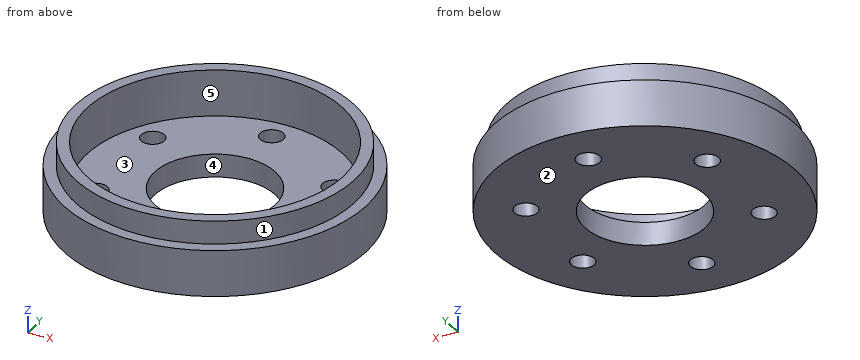
from build123d import *

# Parameters (mm, degrees)
SKETCH_1_R          = 32.5
SKETCH_1_R_2        = 13
EXTRUDE_1_DEPTH     = 5
SKETCH_2_R          = 32.5
SKETCH_2_R_2        = 27.5
EXTRUDE_2_DEPTH     = 5
SKETCH_3_R          = 2.5
CUT_EXTRUDE_1_DEPTH = 47.233105022
SKETCH_4_R          = 30
SKETCH_4_R_2        = 27.5
EXTRUDE_3_DEPTH     = 5


with BuildPart() as part:
    # 草图1 → 凸台-拉伸1 (new body)
    with BuildSketch(Plane.XY):
        Circle(SKETCH_1_R)
        Circle(SKETCH_1_R_2, mode=Mode.SUBTRACT)
    extrude(amount=EXTRUDE_1_DEPTH)

    # 草图2 → 凸台-拉伸2 (add)
    with BuildSketch(Plane.XY.offset(5)):
        Circle(SKETCH_2_R)
        Circle(SKETCH_2_R_2, mode=Mode.SUBTRACT)
    extrude(amount=EXTRUDE_2_DEPTH)

    # 草图3 → 切除-拉伸1 (cut, through all)
    with BuildSketch(Plane.XY.offset(5)):
        with Locations((0, 22.5)):
            Circle(SKETCH_3_R)
        with Locations((19.485571585, 11.25)):
            Circle(SKETCH_3_R)
        with Locations((19.485571585, -11.25)):
            Circle(SKETCH_3_R)
        with Locations((0, -22.5)):
            Circle(SKETCH_3_R)
        with Locations((-19.485571585, -11.25)):
            Circle(SKETCH_3_R)
        with Locations((-19.485571585, 11.25)):
            Circle(SKETCH_3_R)
    extrude(amount=-CUT_EXTRUDE_1_DEPTH, mode=Mode.SUBTRACT)

    # 草图4 → 凸台-拉伸3 (add)
    with BuildSketch(Plane.XY.offset(10)):
        Circle(SKETCH_4_R)
        Circle(SKETCH_4_R_2, mode=Mode.SUBTRACT)
    extrude(amount=EXTRUDE_3_DEPTH)


solid = part.part
Input: part model. Units: mm. Frame: model coordinates. Face numbers are marked on the shaded views. A direction names the side the tool comes from. Round coordinates to 2 decimals unless told otherwise and drop trailing zeros. Order: outer loops, then holes, each group sorted by start corner. A loop starts at its lowest first (then second) coordinate and runs counter-clockwise, first axis right, second up. Notation, with made-up numbers: (12.5, -17.75) - (68.5, -17.75) arc R12 cw to (68.5, -9.75) - close; hole circle Ø4 at (34.25, 72.5). An arc over 180 degrees is marked (long way). Use a Markdown table: item, result.
1. Material intervals for probe 1 along Y at (x, z) = (0, 1.8); probe 2 along Y at (x, z) = (0, 9.75); probe 3 along Y at (x, z) = (0.5, 12.75), sorted ascending.
Evaluation:
| item | result |
|---|---|
| probe 1 | -32.5 to -25, -20 to -13, 13 to 20, 25 to 32.5 |
| probe 2 | -32.5 to -27.5, 27.5 to 32.5 |
| probe 3 | -30 to -27.5, 27.5 to 30 |
2. Section B-B on y = 0. Return the cut outline in (x, z).
Evaluation:
| item | result |
|---|---|
| outline | (-32.5, 0) - (-13, 0) - (-13, 5) - (-27.5, 5) - (-27.5, 15) - (-30, 15) - (-30, 10) - (-32.5, 10) - close; (13, 0) - (32.5, 0) - (32.5, 10) - (30, 10) - (30, 15) - (27.5, 15) - (27.5, 5) - (13, 5) - close |
3. Section C-C on z = 3.25. Return the cut outline in (x, y).
Evaluation:
| item | result |
|---|---|
| outline | circle Ø65 at (0, 0); hole circle Ø5 at (-19.49, -11.25); hole circle Ø5 at (-19.49, 11.25); hole circle Ø26 at (0, 0); hole circle Ø5 at (0, -22.5); hole circle Ø5 at (0, 22.5); hole circle Ø5 at (19.49, -11.25); hole circle Ø5 at (19.49, 11.25) |
4. Access query for the marked faces 4 and 5. Directions: +Z, -Z, +X, -X, +Y, -Y. A direction counts if a zero-diameter tool reaches every point of the face in a straight line with its end or side. Return the directions, or none.
Evaluation:
| item | result |
|---|---|
| face 4 | +Z, -Z |
| face 5 | +Z |
5. Section D-D on x = -8.5. Return the cut outline in (y, z).
Evaluation:
| item | result |
|---|---|
| outline | (-31.37, 0) - (-9.84, 0) - (-9.84, 5) - (-26.15, 5) - (-26.15, 15) - (-28.77, 15) - (-28.77, 10) - (-31.37, 10) - close; (9.84, 0) - (31.37, 0) - (31.37, 10) - (28.77, 10) - (28.77, 15) - (26.15, 15) - (26.15, 5) - (9.84, 5) - close |
6. First-contact query: pin 1 (2 mm diameter, centred on y = 21.5, z = 2, fed in from +X); pin 2 (16.5 mm diameter, centred on x = 12.5, y = 0, fed in from +Z); pin 3 (6 mm diameter, centred on x = -15.5, z = 4, fed in from +Y). Flat tips, straight axial feed; report the tip coordinate or a pass-through.
Evaluation:
| item | result |
|---|---|
| pin 1 | x = 25.22 |
| pin 2 | z = 5 |
| pin 3 | y = 30 |
7. Section A-A on x = 0. Return the cut outline in (y, z).
Evaluation:
| item | result |
|---|---|
| outline | (-32.5, 0) - (-25, 0) - (-25, 5) - (-27.5, 5) - (-27.5, 15) - (-30, 15) - (-30, 10) - (-32.5, 10) - close; (-20, 0) - (-13, 0) - (-13, 5) - (-20, 5) - close; (13, 0) - (20, 0) - (20, 5) - (13, 5) - close; (25, 0) - (32.5, 0) - (32.5, 10) - (30, 10) - (30, 15) - (27.5, 15) - (27.5, 5) - (25, 5) - close |
8. Mould query, pull axis X, two halves, no side actions, for the marked faces 1, 2 and 3. Classes: +X half, -X half, draft (parallel to the pull), parting line (faces both ways), or undercut.
Evaluation:
| item | result |
|---|---|
| face 1 | parting line |
| face 2 | draft |
| face 3 | undercut |
